from build123d import *

# Parameters (mm, degrees)
SKETCH1_R           = 12.7
BOSS_EXTRUDE1_DEPTH = 3.175
SKETCH2_R           = 12.7
BOSS_EXTRUDE2_DEPTH = 6.35


with BuildPart() as part:
    # Sketch1 → Boss-Extrude1 (new body)
    with BuildSketch(Plane.XY):
        Polygon((-323.85, -25.4), (-25.546675569, -25.4), (-25.546675569, -76.2), (25.253324431, -76.2), (25.253324431, -25.4), (323.85, -25.4), (323.85, 25.4), (-323.85, 25.4), align=None)
        with Locations((0, -48.981872029)):
            Circle(SKETCH1_R, mode=Mode.SUBTRACT)
    extrude(amount=BOSS_EXTRUDE1_DEPTH)

    # Sketch2 → Boss-Extrude2 (add)
    with BuildSketch(Plane.XY.offset(3.175)):
        with Locations(Location((296.914396716, 0, 0), (0, 0, 180))):
            Circle(SKETCH2_R)
    extrude(amount=BOSS_EXTRUDE2_DEPTH)


solid = part.part
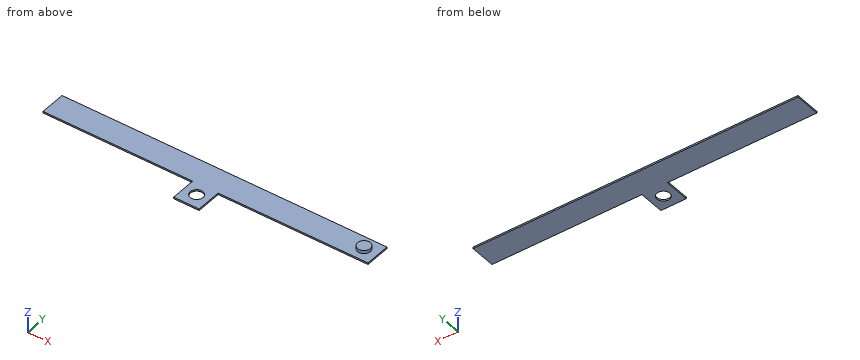
Source: CAD feature listing. Evaluate the final solid. Frame: model axes, mm. Give positions to 0.01 mm unless a question says otherwise; leave off trailing zeros. Order: outer loops, then holes, each group sorted by start corner. A loop starts at its lowest first (then second) coordinate and runs counter-clockwise, first axis right, second up. Notation, with made-up numbers: (9.25, 40) -> (21.25, 40) arc R17 ccw to (21.25, 48) -> close; hole circle Ø9 at (44.5, 54.5). An arc over 180 degrees is marked (long way). Write item = value, one per line.
Q1. Cut plane D-D, the plane x = 166. Output: boundary loops of the cut face in (y, z) (3 decimals), and give its area (3 significant figures).
Data:
outline = (-25.4, 0) -> (25.4, 0) -> (25.4, 3.175) -> (-25.4, 3.175) -> close
area = 161 mm^2
Q2. Material intervals for line 1 (Y direction, x = 0, z = 2.2); line 2 (Z direction, x = 160.5, y = 7) (3 decimals); line 3 (X direction, y = -37.5, z = 2.5), sorted ascending. Write a range as from..to.
Data:
line_1 = -76.2..-61.68, -36.28..25.4
line_2 = 0..3.175
line_3 = -25.55..-5.43, 5.43..25.25
Q3. Pin query (flat end, axial travel): pin 1 (15 mm diameter, centred on x = 0, y = -48.98, fed in from +Z); pin 2 (1 mm diameter, centred on y = -39, z = 1.5, fed in from +X); pin 3 (1.6 mm diameter, centred on y = -61.5, z = 1.5, fed in from -X); pin 4 (1.6 mm diameter, centred on x = 218, z = 1.5, fed in from -Y). Return the tip coordinate at first contact, or that it passes through.
Data:
pin_1 = through
pin_2 = 25.25
pin_3 = -25.55
pin_4 = -25.4
Q4. Cut plane A-A, the plane x = 0. Output: boundary loops of the cut face in (y, z) (3 decimals).
Data:
outline = (-76.2, 0) -> (-61.682, 0) -> (-61.682, 3.175) -> (-76.2, 3.175) -> close; (-36.282, 0) -> (25.4, 0) -> (25.4, 3.175) -> (-36.282, 3.175) -> close
Q5. Cut plane C-C, the plane y = 19. Output: boundary loops of the cut face in (x, z) (3 decimals).
Data:
outline = (-323.85, 0) -> (323.85, 0) -> (323.85, 3.175) -> (-323.85, 3.175) -> close
Q6. Cut plane B-B, the plane z = 6.75. Output: boundary loops of the cut face in (x, y).
Data:
outline = circle Ø25.4 at (296.91, 0)
